```python
from build123d import *

# Parameters (mm, degrees)
CROQUIS1_W              = 42.3
CROQUIS1_H              = 42.3
SALIENTE_EXTRUIR1_DEPTH = 12
CORTAR_EXTRUIR1_DEPTH   = 2
CHAFL_N1_SIZE           = 2
CROQUIS3_R              = 2.5
CORTAR_EXTRUIR2_DEPTH   = 11


with BuildPart() as part:
    # Croquis1 → Saliente-Extruir1 (new body)
    with BuildSketch(Plane(origin=(0, 0, 0), x_dir=(1, 0, 0), z_dir=(0, 1, 0))):
        Rectangle(CROQUIS1_W, CROQUIS1_H)
    extrude(amount=SALIENTE_EXTRUIR1_DEPTH)

    # Croquis2 → Cortar-Extruir1 (cut)
    with BuildSketch(Plane(origin=(0, 12, 0), x_dir=(1, 0, 0), z_dir=(0, 1, 0))):
        with BuildLine():
            Line((-21.15, 13.329572386), (-21.15, -13.329572386))
            ThreePointArc((-21.15, -13.329572386), (-17.67766953, -17.67766953), (-13.329572386, -21.15))
            Line((-13.329572386, -21.15), (13.329572386, -21.15))
            ThreePointArc((13.329572386, -21.15), (17.67766953, -17.67766953), (21.15, -13.329572386))
            Line((21.15, -13.329572386), (21.15, 13.329572386))
            ThreePointArc((21.15, 13.329572386), (17.67766953, 17.67766953), (13.329572386, 21.15))
            Line((13.329572386, 21.15), (-13.329572386, 21.15))
            ThreePointArc((-13.329572386, 21.15), (-17.67766953, 17.67766953), (-21.15, 13.329572386))
        make_face()
    extrude(amount=-CORTAR_EXTRUIR1_DEPTH, mode=Mode.SUBTRACT)

    # Chaflán1
    chafl_n1_edges = [part.edges().sort_by_distance(p)[0] for p in [
        (21.15, 6, 21.15),
        (-21.15, 6, 21.15),
        (-21.15, 6, -21.15),
        (21.15, 6, -21.15),
    ]]
    chamfer(chafl_n1_edges, length=CHAFL_N1_SIZE)

    # Croquis3 → Cortar-Extruir2 (cut, through all)
    with BuildSketch(Plane(origin=(0, 10, 0), x_dir=(1, 0, 0), z_dir=(0, 1, 0))):
        Circle(CROQUIS3_R)
    extrude(amount=-CORTAR_EXTRUIR2_DEPTH, mode=Mode.SUBTRACT)


solid = part.part
```
For this review, take the finished solid that the model builds, in its own axes (mm). A direction names the side the tool comes from. Coordinates: 2 decimals unless noted, no trailing zeros. Write each loop counter-clockwise with the first axis right and the second up, starting at its lowest first coordinate (ties: lowest second). Pieces come first, ordered by that corner, then holes.
(1) For pin 1 Ø6.5 at (x, z) = (0, 0) entering from -Y, flat-tipped, find the tip position at first contact; note if it passes through.
(2) Tool access review of faces 1 (the face through (0, 10, -5)), 2 (the face through (-18, 12, 18)): name each direction out of +Z, -Z, +X, -X, +Y, -Y from which nothing blocks a thin tool from reaching the whole face with its end or side.
(3) Add section C-C on x = 0. Give the boundary of the cut face in (y, z).
(4) The part is to be moulded in two halves that separate along Z. For faces 3 (the face through (20.2, 5.9, 20.1)), 4 (the face through (-0.54, 5.07, 2.44)), 5 (the face through (21.15, 6, 0)), say which applies: +Z half, -Z half, draft (parallel to the pull), parting line (faces both ways), or undercut.
(5) Add section D-D on z = 16.5. Give the boundary of the cut face in (x, y).
(6) Add section B-B on y = 5.5. Give the boundary of the cut face in (x, z).
(7) Add section A-A on z = 0. Give the boundary of the cut face in (x, y).
(8) Wall thickness on probe 1 along X at (y, z) = (2.5, 0); probe 2 along Y at (x, z) = (14, -17): over which ranges is each line inside the solid? List them lowest first.
Answer sheet:
1. pin 1: stops at y = 0
2. face 1: +Y
2. face 2: +Z, -Z, +X, -X, +Y
3. outline: (0, -21.15) - (10, -21.15) - (10, -2.5) - (0, -2.5) - close; (0, 2.5) - (10, 2.5) - (10, 21.15) - (0, 21.15) - close
4. face 3: +Z half
4. face 4: undercut
4. face 5: draft
5. outline: (-21.15, 0) - (21.15, 0) - (21.15, 12) - (18.78, 12) - (18.78, 10) - (-18.78, 10) - (-18.78, 12) - (-21.15, 12) - close
6. outline: (-21.15, -19.15) - (-19.15, -21.15) - (19.15, -21.15) - (21.15, -19.15) - (21.15, 19.15) - (19.15, 21.15) - (-19.15, 21.15) - (-21.15, 19.15) - close; hole circle Ø5 at (0, 0)
7. outline: (-21.15, 0) - (-2.5, 0) - (-2.5, 10) - (-21.15, 10) - close; (2.5, 0) - (21.15, 0) - (21.15, 10) - (2.5, 10) - close
8. probe 1: x = -21.15 to -2.5, 2.5 to 21.15
8. probe 2: y = 0 to 10
